Drawing for the job (mm, zero at the part's lowest x, y, z). Give positions to 0.01 mm unless a question says otherwise; leave off trailing zeros. Order: outer loops, then holes, each group sorted by start corner. A loop starts at its lowest first (then second) coordinate and runs counter-clockwise, first axis right, second up. Notation, with made-up numbers: M 21.5,-9 L 65.5,-9 A22 ccw 65.5,-3 Z; hole C 43,75.25 d8. An arc over 180 degrees is marked long. One line per item, written item: value.
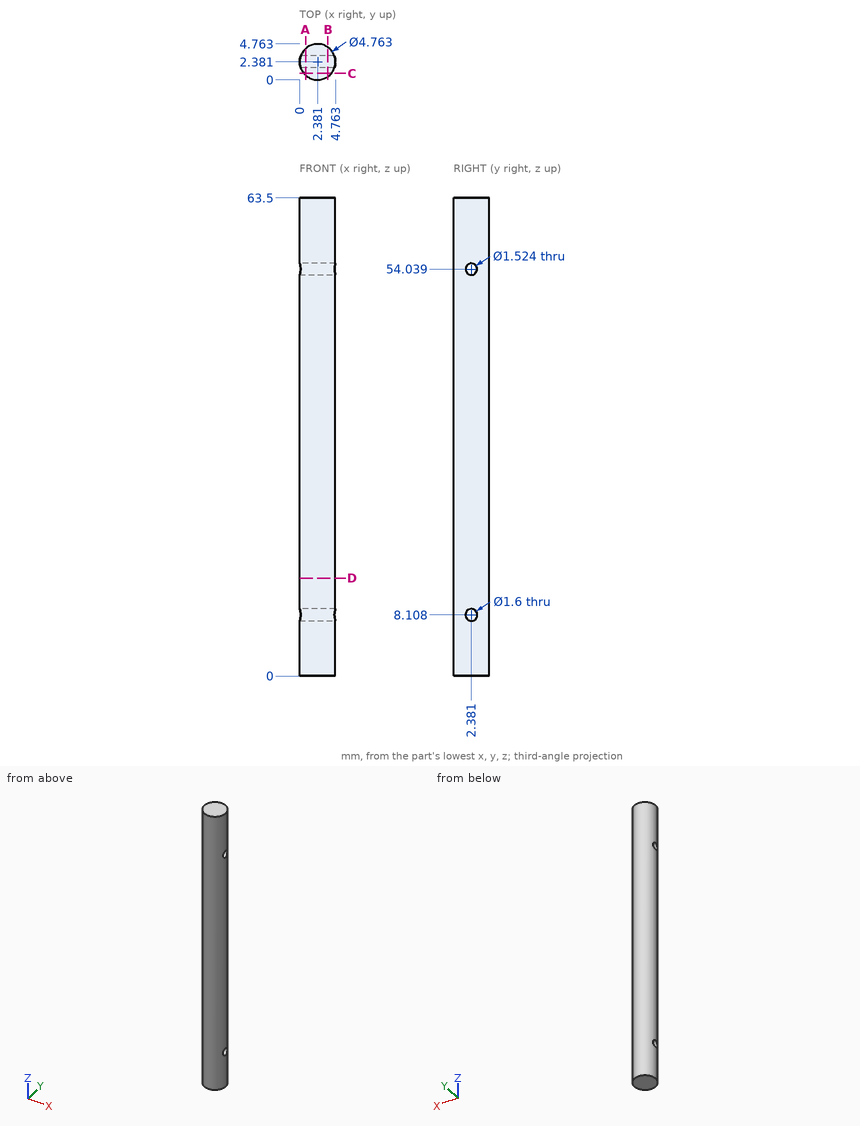
1) Saw through at B-B, the plane x = 3.75. Write the cut outline in (y, z) (1 decimal).
Check values:
outline: M 0.4,0 L 4.3,0 L 4.3,63.5 L 0.4,63.5 Z; hole C 2.4,8.1 d1.6; hole C 2.4,54 d1.5
2) Saw through at D-D, the plane z = 13. Write the cut outline in (x, y), then the cut area to 3 significant figures.
Check values:
outline: C 2.38,2.38 d4.76
area: 17.8 mm^2
3) Saw through at A-A, the plane x = 0.8. Write the cut outline in (y, z) (1 decimal), then the cut area to 3 significant figures.
Check values:
outline: M 0.6,0 L 4.2,0 L 4.2,63.5 L 0.6,63.5 Z; hole C 2.4,8.1 d1.6; hole C 2.4,54 d1.5
area: 222 mm^2
4) Saw through at C-C, the plane y = 0.85. Write the cut outline in (x, z) (1 decimal).
Check values:
outline: M 0.6,0 L 4.2,0 L 4.2,63.5 L 0.6,63.5 Z
5) Drill centre lines: probe 1 along Z at (x, y) = (2.75, 2.5) (1 decimal); probe 2 along Z at (x, y) = (0.7, 1.85) (1 decimal); probe 3 along X at (y, z) = (2.6, 52.5). Where is each one in solid material? Low to high. Write a range as from..to.
Check values:
probe 1: 0..7.3, 8.9..53.3, 54.8..63.5
probe 2: 0..7.5, 8.7..53.5, 54.6..63.5
probe 3: 0.01..4.75
6) Pin check, flat tips, straight feed: pin 1 (1 mm diameter, centred on x = 4, z = 23.5, fed in from +Y); pin 2 (1.5 mm diameter, centred on x = 3.5, z = 33, fed in from +Y). Stop position of each tip, or through.
Check values:
pin 1: y = 4.48
pin 2: y = 4.73
